Build history of the part. All positions in model axes, mm. Face numbers are marked on the shaded views. A direction names the side the tool comes from. Round coordinates to 2 decimals unless told otherwise and drop trailing zeros. Write each loop counter-clockwise with the first axis right and the second up, starting at its lowest first coordinate (ties: lowest second). Pieces come first, ordered by that corner, then holes.
Item 1: Drop flat-ended pins along their axis: pin 1 Ø1.7 at (y, z) = (19.5, -4) entering from -X; pin 2 Ø3 at (x, y) = (-31, -32) entering from -Z; pin 3 Ø4.5 at (x, y) = (-17.5, 8) entering from -Z. Give the stop position or say it passes through.
Item 2: Band-saw the part on B-B, the plane y = -31.5. Write the cut outline in (x, z) (3 decimals), then the cut area to 3 significant figures.
Item 3: Wall check: probe 1 along X at (y, z) = (26, 2.25) (3 decimals); probe 2 along Y at (x, z) = (-20.5, -2.5) (3 decimals); probe 3 along Z at (x, y) = (-13.5, -14.5). Give the ranges that are in metal, low to high.
Item 4: Band-saw the part on D-D, the plane z = 2.5. Write the cut outline in (x, y) (3 decimals), then the cut area to 3 significant figures.
Item 5: 3-axis set-ups, long thin cutter, end or side, ignore diameter. For the marked faces 1, 2, 3 and 4: which of +Z, -Z, +X, -X, +Y, -Y reach the whole face in a straight line?
Item 6: Band-saw the part on C-C, the plane x = 20. Write the cut outline in (y, z) (3 decimals).
Item 7: Band-saw the part on A-A, the plane z = -6.25. Write the cut outline in (x, y) (3 decimals), then the cut area to 3 significant figures.
```python
from build123d import *

# Parameters (mm, degrees)
SKETCH_1_W          = 70.09
SKETCH_1_H          = 70.09
EXTRUDE_1_DEPTH     = 5
SKETCH_2_R          = 1.8
EXTRUDE_2_DEPTH     = 10
SKETCH_4_W          = 57
SKETCH_4_H          = 5
CUT_EXTRUDE_2_DEPTH = 15
SKETCH_5_W          = 56.8
SKETCH_5_H          = 1.545
EXTRUDE_3_DEPTH     = 12
SKETCH_6_W          = 6
SKETCH_6_H          = 18
EXTRUDE_4_DEPTH     = 3.7
SKETCH_7_W          = 15
SKETCH_7_H          = 20
EXTRUDE_5_DEPTH     = 2


with BuildPart() as part:
    # 草图1 → 凸台-拉伸1 (new body)
    with BuildSketch(Plane.XY):
        Rectangle(SKETCH_1_W, SKETCH_1_H)
    extrude(amount=EXTRUDE_1_DEPTH)

    # 草图2 → 凸台-拉伸2 (add)
    with BuildSketch(Plane.XY):
        with Locations((31.5, 31.5)):
            Circle(SKETCH_2_R)
        with Locations((31.5, -31.5)):
            Circle(SKETCH_2_R)
        with Locations((-31.5, -31.5)):
            Circle(SKETCH_2_R)
        with Locations((-31.5, 31.5)):
            Circle(SKETCH_2_R)
    extrude(amount=-EXTRUDE_2_DEPTH)

    # 草图4 → 切除-拉伸2 (cut)
    with BuildSketch(Plane(origin=(0, 35.045, 0), x_dir=(1, 0, 0), z_dir=(0, 1, 0))):
        with Locations((0, -2.5)):
            Rectangle(SKETCH_4_W, SKETCH_4_H)
    extrude(amount=-CUT_EXTRUDE_2_DEPTH, mode=Mode.SUBTRACT)

    # 草图5 → 凸台-拉伸3 (add)
    with BuildSketch(Plane(origin=(0, 0, 0), x_dir=(-1, 0, 0), z_dir=(0, 0, -1))):
        with Locations((0, 19.2725)):
            Rectangle(SKETCH_5_W, SKETCH_5_H)
    extrude(amount=EXTRUDE_3_DEPTH)

    # 草图6 → 凸台-拉伸4 (add)
    with BuildSketch(Plane(origin=(0, 0, 0), x_dir=(-1, 0, 0), z_dir=(0, 0, -1))):
        with Locations((-19.5, 9.5)):
            Rectangle(SKETCH_6_W, SKETCH_6_H)
    extrude(amount=EXTRUDE_4_DEPTH)

    # 草图7 → 凸台-拉伸5 (add)
    with BuildSketch(Plane(origin=(0, 0, 0), x_dir=(-1, 0, 0), z_dir=(0, 0, -1))):
        with Locations((15.5, 8.5)):
            Rectangle(SKETCH_7_W, SKETCH_7_H)
    extrude(amount=EXTRUDE_5_DEPTH)


solid = part.part
```
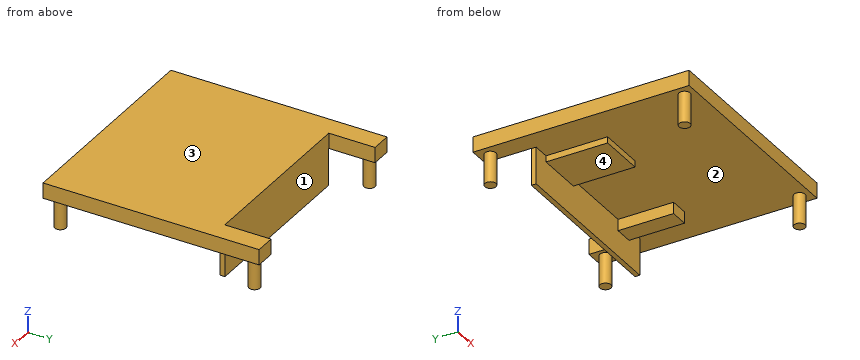
Results:
1. pin 1: stops at x = -28.4
1. pin 2: stops at z = -10
1. pin 3: stops at z = -2
2. outline: (-35.045, 0) - (-33.3, 0) - (-33.3, -10) - (-29.7, -10) - (-29.7, 0) - (29.7, 0) - (29.7, -10) - (33.3, -10) - (33.3, 0) - (35.045, 0) - (35.045, 5) - (-35.045, 5) - close
2. area: 422 mm2
3. probe 1: x = -35.045 to -28.5, 28.5 to 35.045
3. probe 2: y = 18.5 to 20.045
3. probe 3: z = 0 to 5
4. outline: (-35.045, -35.045) - (35.045, -35.045) - (35.045, 35.045) - (28.5, 35.045) - (28.5, 20.045) - (-28.5, 20.045) - (-28.5, 35.045) - (-35.045, 35.045) - close
4. area: 4,060 mm2
5. face 1: +Z, -Z, +Y
5. face 2: -Z
5. face 3: +Z, +X, -X, +Y, -Y
5. face 4: -Z, -X, -Y
6. outline: (-35.045, 0) - (0.5, 0) - (0.5, -3.7) - (18.5, -3.7) - (18.5, -12) - (20.045, -12) - (20.045, 5) - (-35.045, 5) - close
7. outline: circle Ø3.6 at (-31.5, -31.5); circle Ø3.6 at (-31.5, 31.5); (-28.4, 18.5) - (28.4, 18.5) - (28.4, 20.045) - (-28.4, 20.045) - close; circle Ø3.6 at (31.5, -31.5); circle Ø3.6 at (31.5, 31.5)
7. area: 128 mm2
